Geometry: final body of the model. Coordinates: model frame, mm. A direction names the side the tool comes from. Give positions to 0.01 mm unless a question says otherwise; leave off trailing zeros. Order: outer loops, then holes, each group sorted by start corner. A loop starts at its lowest first (then second) coordinate and runs counter-clockwise, first axis right, second up. Notation, with made-up numbers: (67.5, -13) -> (105.5, -13) arc R34 ccw to (105.5, 17) -> close; hole circle Ø4 at (15.5, 35). An arc over 180 degrees is marked (long way). One line per question, with ' | ' between items. Start each with the question number.
(1) Ray query, L1, parallel to Y at x = 96, z = 78 (3 decimals); L2, parallel to X at y = 27.5, z = 132; L3, parallel to Z at x = -112.5, y = -12.5. Return the intervals inside material, ascending.
(2) Set-up query: faces 1 (the face through (145.89, -2, 123)), 2 (the face through (-2, -107.315, 128)). Return all of +Z, -Z, +X, -X, +Y, -Y with unobstructed straight access to the full face (end or side cutting, diameter ignored); none if empty.
(3) First-contact query: pin 1 Ø8 at (x, y) = (-19.5, 40) entering from +Z. Flat tip, straight axial feed; report the tip coordinate or a pass-through.
(4) Section A-A (z = 84). Return loops of the section in (x, y) (3 decimals).
(5) Mould query, pull axis Y, two halves, no side actions, for faces 3 (the face through (-145.89, -2, 123)), 4 (the face through (-2, 107.315, 128)), 5 (the face through (-2, -117.315, 123)). Classes: +Y half, -Y half, draft (parallel to the pull), parting line (faces both ways), or undercut.
```python
from build123d import *

# Parameters (mm, degrees)
CROQUIS1_W              = 291.78
CROQUIS1_H              = 234.63
CROQUIS1_W_2            = 271.78
CROQUIS1_H_2            = 214.63
SALIENTE_EXTRUIR1_DEPTH = 250
CROQUIS2_W              = 291.78
CROQUIS2_H              = 234.63
SALIENTE_EXTRUIR2_DEPTH = 10
REDONDEO1_R             = 5


with BuildPart() as part:
    # Croquis1 → Saliente-Extruir1 (new body)
    with BuildSketch(Plane.XY):
        Rectangle(CROQUIS1_W, CROQUIS1_H)
        Rectangle(CROQUIS1_W_2, CROQUIS1_H_2, mode=Mode.SUBTRACT)
    extrude(amount=SALIENTE_EXTRUIR1_DEPTH)

    # Croquis2 → Saliente-Extruir2 (add)
    with BuildSketch(Plane.XY):
        Rectangle(CROQUIS2_W, CROQUIS2_H)
    extrude(amount=SALIENTE_EXTRUIR2_DEPTH)

    # Redondeo1
    redondeo1_edges = [part.edges().sort_by_distance(p)[0] for p in [
        (145.89, 0, 250),
        (-135.89, 107.315, 130),
        (-135.89, -107.315, 130),
        (135.89, -107.315, 130),
        (135.89, 107.315, 130),
        (-135.89, 0, 250),
        (0, 117.315, 250),
        (0, -107.315, 250),
        (135.89, 0, 250),
        (0, 107.315, 250),
        (0, 107.315, 10),
        (-135.89, 0, 10),
        (0, -107.315, 10),
        (135.89, 0, 10),
        (-145.89, 0, 250),
        (0, 117.315, 0),
        (145.89, 0, 0),
        (0, -117.315, 0),
        (-145.89, 0, 0),
        (-145.89, 117.315, 125),
        (145.89, 117.315, 125),
        (145.89, -117.315, 125),
        (-145.89, -117.315, 125),
        (0, -117.315, 250),
    ]]
    fillet(redondeo1_edges, radius=REDONDEO1_R - 0.0001)  # a hair under: the kernel refuses the full size


solid = part.part
```
Response:
1) L1: y = -117.315 to -107.315, 107.315 to 117.315 | L2: x = -145.89 to -135.89, 135.89 to 145.89 | L3: z = 0 to 10
2) face 1: +Z, -Z, +X, +Y, -Y | face 2: +Z
3) pin 1: stops at z = 10
4) outline: (-145.89, -112.315) arc R5 ccw to (-140.89, -117.315) -> (140.89, -117.315) arc R5 ccw to (145.89, -112.315) -> (145.89, 112.315) arc R5 ccw to (140.89, 117.315) -> (-140.89, 117.315) arc R5 ccw to (-145.89, 112.315) -> close; hole (-135.89, -102.315) arc R5 ccw to (-130.89, -107.315) -> (130.89, -107.315) arc R5 ccw to (135.89, -102.315) -> (135.89, 102.315) arc R5 ccw to (130.89, 107.315) -> (-130.89, 107.315) arc R5 ccw to (-135.89, 102.315) -> close
5) face 3: draft | face 4: undercut | face 5: -Y half
